Model file for the job. Use its own axes, mm. Give positions to 0.01 mm unless a question says otherwise; leave off trailing zeros. Write each loop counter-clockwise with the first axis right and the second up, starting at its lowest first coordinate (ties: lowest second). Pieces come first, ordered by that corner, then holes. Notation, with made-up numbers: (-26, 16.5) - (-7, 16.5) arc R7 cw to (-7, 22.5) - close; hole circle Ø9 at (52.5, 70.5). An arc over 180 degrees is marked (long way). Use a Markdown table: item, result. Add a question column.
Autodesk Inventor part; units mm, degrees
ref_plane "YZ Plane" through (0, 0, 0) normal (1, 0, 0) x (0, 1, 0)
ref_plane "XZ Plane" through (0, 0, 0) normal (0, 1, 0) x (-1, 0, 0)
ref_plane "XY Plane" through (0, 0, 0) normal (0, 0, 1) x (1, 0, 0)
sketch "Sketch1" plane through (0, 0, 0) normal (0, 1, 0) x (-1, 0, 0)
  line L0 (-34.4, 69.4) -> (34.4, 69.4)
  line L1 (34.4, 69.4) -> (34.4, -69.4)
  line L2 (34.4, -69.4) -> (-34.4, -69.4)
  line L3 (-34.4, -69.4) -> (-34.4, 69.4)
  line L4 (-34.4, 69.4) -> (34.4, -69.4) construction
  line L5 (34.4, 69.4) -> (-34.4, -69.4) construction
  line L6 (32.4, -67.4) -> (32.4, 67.4)
  line L7 (32.4, 67.4) -> (-32.4, 67.4)
  line L8 (-32.4, 67.4) -> (-32.4, -67.4)
  line L9 (-32.4, -67.4) -> (32.4, -67.4)
  point P0 (0, 0)
  dimension "d0" = 68.8
  dimension "d1" = 138.8
  dimension "d2" = 2
extrude "Extrusion1" add sketch "Sketch1" along normal blind 10
sketch "Sketch2" plane through (0, 0, 0) normal (0, -1, 0) x (1, 0, 0)
  line L0 (-49.4, 84.4) -> (49.4, 84.4)
  line L1 (49.4, 84.4) -> (49.4, -84.4)
  line L2 (49.4, -84.4) -> (-49.4, -84.4)
  line L3 (-49.4, -84.4) -> (-49.4, 84.4)
  line L4 (-49.4, 84.4) -> (49.4, -84.4) construction
  line L5 (49.4, 84.4) -> (-49.4, -84.4) construction
  line L6 (34.4, 69.4) -> (34.4, -69.4)
  line L7 (-34.4, 69.4) -> (34.4, 69.4)
  line L8 (34.4, -69.4) -> (-34.4, -69.4)
  line L9 (-34.4, -69.4) -> (-34.4, 69.4)
  point P0 (0, 0)
  dimension "d5" = 15
  dimension "d6" = 15
extrude "Extrusion2" add sketch "Sketch2" against normal blind 2
fillet "Fillet1" radius 4 4 edges at (49.4, 1, -84.4) (49.4, 1, 84.4) (-49.4, 1, 84.4) (-49.4, 1, -84.4)
sketch "Sketch3" plane through (0, 0, 0) normal (0, -1, 0) x (1, 0, 0)
  arc A0 (-49.4, -80.4) -> (-45.4, -84.4) centre (-45.4, -80.4) ccw
  line L0 (-49.4, 80.4) -> (-49.4, -80.4)
  arc A1 (-45.4, 84.4) -> (-49.4, 80.4) centre (-45.4, 80.4) ccw
  line L1 (45.4, 84.4) -> (-45.4, 84.4)
  arc A2 (49.4, 80.4) -> (45.4, 84.4) centre (45.4, 80.4) ccw
  line L2 (49.4, -80.4) -> (49.4, 80.4)
  arc A3 (45.4, -84.4) -> (49.4, -80.4) centre (45.4, -80.4) ccw
  line L3 (-45.4, -84.4) -> (45.4, -84.4)
  line L4 (34.4, 69.4) -> (45.4, 80.4)
  circle A4 centre (39.9, 74.9) radius 2.75
  line L5 (34.4, -69.4) -> (-34.4, -69.4)
  line L6 (34.4, -69.4) -> (45.4, -80.4)
  circle A5 centre (39.9, -74.9) radius 2.75
  line L7 (45.4, -84.4) -> (-45.4, -84.4)
  line L8 (0, -84.4) -> (0, -77.4)
  circle A6 centre (-39.9, 74.9) radius 2.75
  circle A7 centre (-39.9, -74.9) radius 2.75
  point P0 (32.4, -67.4)
  point P1 (32.4, 67.4)
  point P2 (-32.4, 67.4)
  dimension "d20" = 5.5
  dimension "d21" = 5.5
extrude "Extrusion3" cut sketch "Sketch3" against normal up to surface (2 mm away) contours A4 L4 | L4 A4 | A5 L6 | L6 A5 | A6 | A7
sketch "Sketch4" plane through (0, 2, 0) normal (0, 1, 0) x (1, 0, 0)
  circle A0 centre (-39.9, -74.9) radius 2.75
  circle A1 centre (-39.9, -74.9) radius 6
  circle A2 centre (39.9, -74.9) radius 2.75
  circle A3 centre (39.9, -74.9) radius 6
  line L0 (33.9209, -74.4) -> (-33.9209, -74.4)
  line L1 (-34.4, -69.4) -> (34.4, -69.4)
  line L2 (0, 0) -> (-15.7082, 0)
  circle A4 centre (-39.9, 74.9) radius 2.75
  circle A5 centre (39.9, 74.9) radius 6
  line L3 (33.9209, 74.4) -> (-33.9209, 74.4)
  circle A6 centre (-39.9, 74.9) radius 6
  line L4 (-39.4, -68.9209) -> (-39.4, 68.9209)
  line L5 (-34.4, 69.4) -> (-34.4, -69.4)
  line L6 (39.4, -68.9209) -> (39.4, 68.9209)
  line L7 (34.4, -69.4) -> (34.4, 69.4)
  circle A7 centre (39.9, 74.9) radius 2.75
  circle A8 centre (-39.9, -74.9) radius 2.75
  circle A9 centre (39.9, -74.9) radius 2.75
  circle A10 centre (-39.9, 74.9) radius 2.75
  arc A11 (-45.4, 84.4) -> (-49.4, 80.4) centre (-45.4, 80.4) ccw
  line L8 (-49.4, 80.4) -> (-49.4, -80.4)
  arc A12 (-49.4, -80.4) -> (-45.4, -84.4) centre (-45.4, -80.4) ccw
  line L9 (-45.4, -84.4) -> (45.4, -84.4)
  arc A13 (45.4, -84.4) -> (49.4, -80.4) centre (45.4, -80.4) ccw
  line L10 (49.4, -80.4) -> (49.4, 80.4)
  arc A14 (49.4, 80.4) -> (45.4, 84.4) centre (45.4, 80.4) ccw
  line L11 (45.4, 84.4) -> (-45.4, 84.4)
  line L12 (34.4, -69.4) -> (34.4, 69.4)
  line L13 (-34.4, -69.4) -> (34.4, -69.4)
  line L14 (-34.4, 69.4) -> (-34.4, -69.4)
  line L15 (34.4, 69.4) -> (-34.4, 69.4)
  dimension "d22" = 12
  dimension "d23" = 12
  dimension "d24" = 5
  dimension "d25" = 5
  dimension "d26" = 5
extrude "Extrusion4" cut sketch "Sketch4" against normal blind 10 contours L11 A14 L10 A13 L9 A12 L8 A11
fillet "Fillet2" radius 4 8 edges at (-39.4, 1, 68.9209) (-33.9209, 1, 74.4) (-33.9209, 1, -74.4) (-39.4, 1, -68.9209) (33.9209, 1, -74.4) (39.4, 1, -68.9209) (39.4, 1, 68.9209) (33.9209, 1, 74.4)
properties part number "_3DPrint"
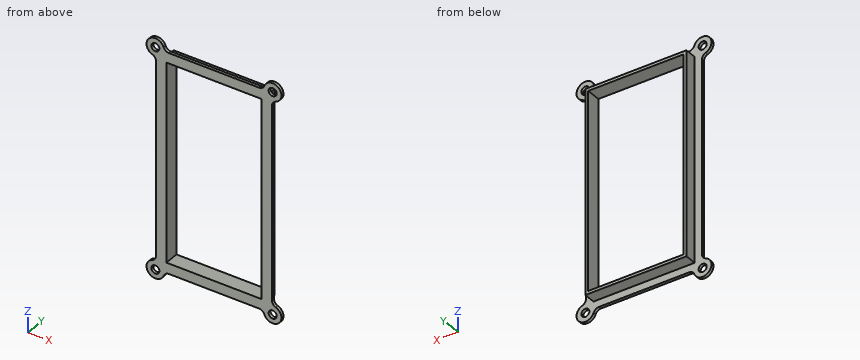
(1) Probe probe 1 along Z at (x, y) = (0, 8.5); probe 2 along X at (y, z) = (3, -38); probe 3 along Z at (x, y) = (39.9, 1.05). List the from-to ranges inside material, lowest first. Write a range as [from, to].
(2) Band-saw the part on B-B (z = 6). Write the cut outline in (x, y), then the cut area to 3 significant figures.
(3) Band-saw the part on C-C (y = 7). Write the cut outline in (x, z).
(4) Flat gauge pins, fed straight in: pin 1 (4 mm diameter, centred on x = -4, y = 7.5, fed in from +Z); pin 2 (2.5 mm diameter, centred on y = 6, z = 20, fed in from -X); pin 3 (0.6 mm diameter, centred on x = 12, y = 1, fed in from -Z). Where does each tip first touch, or does it go through?
(5) Band-saw the part on A-A (x = 10). Write the cut outline in (y, z).
Model answer:
| question | item | result |
|---|---|---|
| 1 | probe 1 | z = [-69.4, -67.4], [67.4, 69.4] |
| 1 | probe 2 | x = [-34.4, -32.4], [32.4, 34.4] |
| 1 | probe 3 | z = [-80.9, -77.65], [-72.15, -67.47], [67.47, 72.15], [77.65, 80.9] |
| 2 | outline | (-39.4, 0) - (-32.4, 0) - (-32.4, 10) - (-34.4, 10) - (-34.4, 2) - (-39.4, 2) - close; (32.4, 0) - (39.4, 0) - (39.4, 2) - (34.4, 2) - (34.4, 10) - (32.4, 10) - close |
| 2 | area | 60.0 mm^2 |
| 3 | outline | (-34.4, -69.4) - (34.4, -69.4) - (34.4, 69.4) - (-34.4, 69.4) - close; hole (-32.4, -67.4) - (32.4, -67.4) - (32.4, 67.4) - (-32.4, 67.4) - close |
| 4 | pin 1 | stops at z = 69.4 |
| 4 | pin 2 | stops at x = -34.4 |
| 4 | pin 3 | stops at z = -74.4 |
| 5 | outline | (0, -74.4) - (2, -74.4) - (2, -69.4) - (10, -69.4) - (10, -67.4) - (0, -67.4) - close; (0, 67.4) - (10, 67.4) - (10, 69.4) - (2, 69.4) - (2, 74.4) - (0, 74.4) - close |
